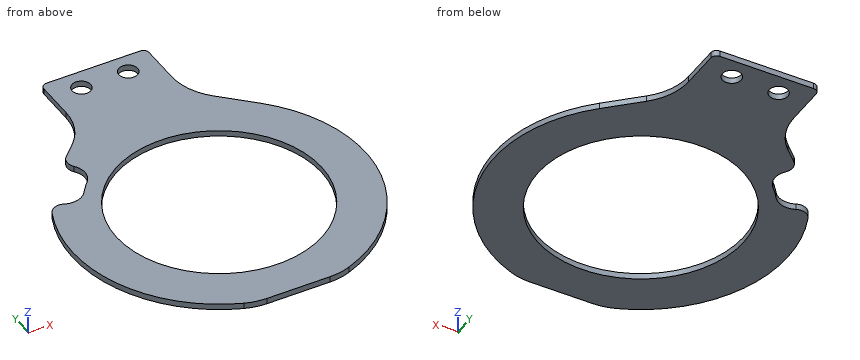
Autodesk Inventor part; units mm, degrees
ref_plane "YZ Plane" through (0, 0, 0) normal (1, 0, 0) x (0, 1, 0)
ref_plane "XZ Plane" through (0, 0, 0) normal (0, 1, 0) x (-1, 0, 0)
ref_plane "XY Plane" through (0, 0, 0) normal (0, 0, 1) x (1, 0, 0)
sketch "Sketch1" plane through (0, 0, 0) normal (0, 0, 1) x (1, 0, 0)
  line L0 (-9, 26) -> (-9, 38)
  line L1 (-9, 38) -> (9, 38)
  line L2 (9, 38) -> (9, 26)
  line L3 (9, 26) -> (17.2958, 18.0514)
  line L4 (-9, 26) -> (-17.2958, 18.0514)
  arc A0 (-17.2958, 18.0514) -> (17.2958, 18.0514) centre (0, 0) ccw
  line L5 (-17.2958, 18.0514) -> (17.2958, 18.0514) construction
  line L6 (-9, 26) -> (9, 26) construction
  circle A1 centre (0, 0) radius 17.5
  point P0 (0, 38)
  dimension "d1" = 38
  dimension "d2" = 18
  dimension "d3" = 50
  dimension "d5" = 35
  dimension "d15" = 12
extrude "Extrusion1" add sketch "Sketch1" along normal blind 1
fillet "Fillet1" radius 10 2 edges at (9, 26, 0.5) (-9, 26, 0.5)
fillet "Fillet2" radius 1 2 edges at (9, 38, 0.5) (-9, 38, 0.5)
sketch "Sketch2" plane through (0, 0, 1) normal (0, 0, 1) x (1, 0, 0)
  circle A0 centre (-4, 34.5) radius 1.6
  circle A1 centre (4, 34.5) radius 1.6
  line L0 (-4, 34.5) -> (4, 34.5) construction
  line L1 (8, 38) -> (-8, 38) construction
  point P0 (0, 0)
  point P1 (0, 34.5)
  dimension "d10" = 3.5
  dimension "d11" = 3.2
  dimension "d12" = 8
extrude "Extrusion2" cut sketch "Sketch2" against normal through all
sketch "Sketch3" plane through (0, 0, 0) normal (0, 0, 1) x (1, 0, 0)
  line L0 (-15, -30) -> (15, -30)
  line L1 (15, -30) -> (15, -24)
  line L2 (15, -24) -> (-15, -24)
  line L3 (-15, -24) -> (-15, -30)
  point P0 (0, 0)
  point P1 (0, -24)
  dimension "d16" = 24
  dimension "d17" = 6
  dimension "d18" = 30
extrude "Trim" cut sketch "Sketch3" along normal through all
fillet "Fillet3" radius 10 2 edges at (7, -24, 0.5) (-7, -24, 0.5)
sketch "Sketch4" plane through (0, 0, 1) normal (0, 0, 1) x (1, 0, 0)
  line L0 (-18.002, 15.1055) -> (18.002, -15.1055) construction
  line L1 (0, 0) -> (14.5661, 0) construction
  arc A0 (-17.0012, 16.2238) -> (-18.9295, 13.9256) centre (0, 0) ccw construction
  arc A1 (-19.3524, 18.4675) -> (-21.5474, 15.8515) centre (0, 0) ccw
  arc A2 (-14.6499, 13.9801) -> (-16.3116, 11.9998) centre (0, 0) ccw
  arc A3 (-14.6499, 13.9801) -> (-19.3524, 18.4675) centre (-17.0012, 16.2238) ccw
  arc A4 (-21.5474, 15.8515) -> (-16.3116, 11.9998) centre (-18.9295, 13.9256) ccw
  dimension "d24" = 40
  dimension "d28" = 47
  dimension "d29" = 6.5
  dimension "d30" = 3
extrude "Extrusion4" cut sketch "Sketch4" against normal through all
fillet "Fillet5" radius 2 2 edges at (-15.9823, 19.31, 0.5) (-21.7544, 12.3186, 0.5)
properties part number "probe-gate" material "Stainless Steel"
The listing builds one solid part. Answer for the finished solid, in the listing's coordinates (mm). Round coordinates to 2 decimals unless told otherwise and drop trailing zeros. Write each loop counter-clockwise with the first axis right and the second up, starting at its lowest first coordinate (ties: lowest second). Pieces come first, ordered by that corner, then holes. Notation, with made-up numbers: (47, -13) -> (73, -13) arc R10 cw to (73, 6) -> close; hole circle Ø3 at (-28.75, 72.5). An arc over 180 degrees is marked (long way). Write item = value, one per line.
1) Given pin 1 (0.5 mm diameter, centred on y = 33.5, z = 0.5, fed in from -X), flat-ended and moving along its own axis, determine where the tip first touches the part or whether it passes through.
Check values:
pin_1 = -9
2) Straight lines are drawn through the part: line 1 along Y through (x, z) = (-4, 0.7); line 2 along Y through (x, z) = (-4.5, 0.5); line 3 along Y through (x, z) = (0, 0.65). For each, find the intervals that lie inside material, in ascending order. Write a range as [from, to].
Check values:
line_1 = [-24, -17.04], [17.04, 32.9], [36.1, 38]
line_2 = [-24, -16.91], [16.91, 32.98], [36.02, 38]
line_3 = [-24, -17.5], [17.5, 38]
3) Section D-D on z = 0.5 is taken. Give the number of separate pieces and of enclosed holes in the cut face, plus the area to 3 significant figures.
Check values:
separate_pieces = 1
enclosed_holes = 3
area = 1,200 mm²
4) Section B-B on x = 0 is taken. Write down the section's boundary in (y, z).
Check values:
outline = (-24, 0) -> (-17.5, 0) -> (-17.5, 1) -> (-24, 1) -> close; (17.5, 0) -> (38, 0) -> (38, 1) -> (17.5, 1) -> close
5) Section A-A on y = 34.5 is taken. Write down the section's boundary in (x, z), plus the area to 3 significant figures.
Check values:
outline = (-9, 0) -> (-5.6, 0) -> (-5.6, 1) -> (-9, 1) -> close; (-2.4, 0) -> (2.4, 0) -> (2.4, 1) -> (-2.4, 1) -> close; (5.6, 0) -> (9, 0) -> (9, 1) -> (5.6, 1) -> close
area = 11.6 mm²
6) Section C-C on y = 0 is taken. Write down the section's boundary in (x, z), plus the area to 3 significant figures.
Check values:
outline = (-25, 0) -> (-17.5, 0) -> (-17.5, 1) -> (-25, 1) -> close; (17.5, 0) -> (25, 0) -> (25, 1) -> (17.5, 1) -> close
area = 15.0 mm²
